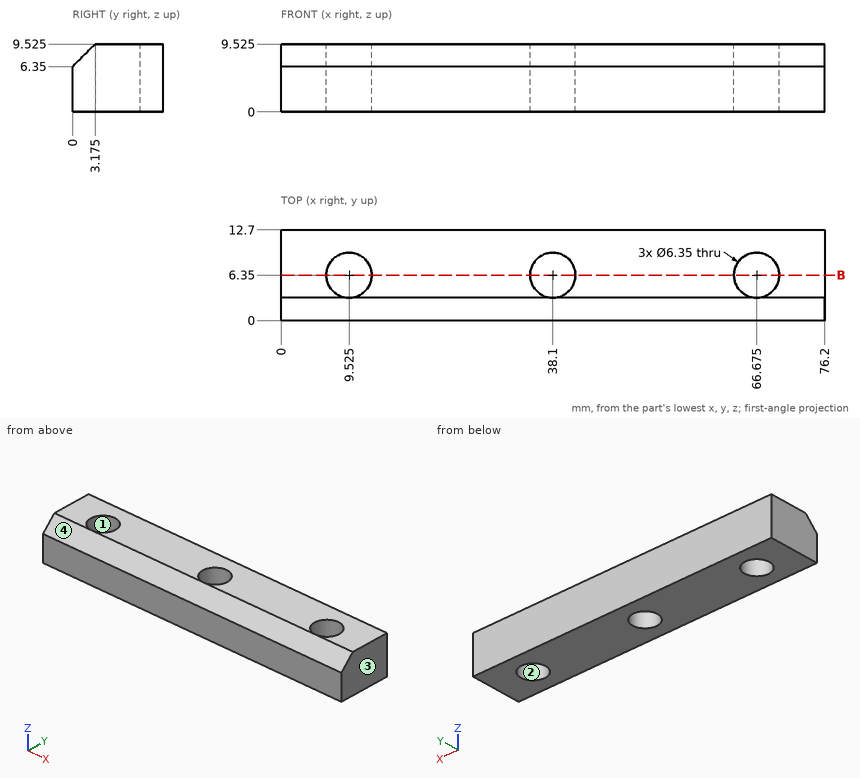
For this review, use the dimensioned drawing (mm, ordinates from the lowest corner) and the shaded views. Round coordinates to 2 decimals unless told otherwise and drop trailing zeros. Answer as a JSON object with one key per item and string values.
(1) Draft analysis for pull direction X (two halves, no side actions). For the marked faces 1, 2, 3 and 4, state which applies: released by +X, released by -X, zero draft, split by the parting line, or undercut.
Resolved:
{"face 1": "undercut", "face 2": "undercut", "face 3": "released by +X", "face 4": "zero draft"}
(2) Take a section at B-B on y = 6.35. Count the separate pieces of the cut face and the enclosed holes in it, and give its area (3 significant figures).
Resolved:
{"separate pieces": "4", "enclosed holes": "0", "area": "544 mm²"}
(3) To check wall thickness, follow line 1 along Y through (x, z) = (38.1, 3.75) (1 decimal); line 2 along X through (y, z) = (6.5, 4); line 3 along X through (y, z) = (3.5, 4.25) (1 decimal). State the ranges of each line that lie inside material, in increasing order.
Resolved:
{"line 1": "0 to 3.2, 9.5 to 12.7", "line 2": "0 to 6.35, 12.7 to 34.93, 41.27 to 63.5, 69.85 to 76.2", "line 3": "0 to 8.1, 10.9 to 36.7, 39.5 to 65.3, 68.1 to 76.2"}
(4) Clearance check with a flat-ended pin moving along its axis: P1, Ø1.5, axis at x = 14.5, y = 6, coming from the -Z side. State where the tip first meets the part, or that it passes through.
Resolved:
{"P1": "z = 0"}
